Geometry check sheet. Reference: the model listing, model coordinates, mm. Face numbers are marked on the shaded views. Give positions to 0.01 mm unless a question says otherwise; leave off trailing zeros. Loops run counter-clockwise (first coordinate to the right, second up) from the corner with the lowest first, then second, coordinate; pieces in that order, holes last. Notation, with made-up numbers: (-31, 89) -> (26, 89) arc R25 ccw to (26, 119) -> close; hole circle Ø10 at (-3.75, 81). An arc over 180 degrees is marked (long way). Write item = value, one per line.
```python
from build123d import *

# Parameters (mm, degrees)
F1_DEPTH = 5.08
F0_W     = 32.385
F0_H     = 5.08
F2_DEPTH = 50.8
F3_DEPTH = 76.2
F4_DEPTH = 127
F5_R     = 2.53999


# Not quite as in the source:
# - a fillet or chamfer is up to 0.001 mm smaller than in the source, because OpenCascade refuses the exact size


with BuildPart() as f1:
    # F0 (on Top) → F1 (new body)
    with BuildSketch(Plane.XY):
        Polygon((23.8125, 15.24), (-23.8125, 15.24), (-23.8125, -15.24), (-16.1925, -15.24), (16.1925, -15.24), (23.8125, -15.24), align=None)
    extrude(amount=F1_DEPTH)

    # F0 (on Top) → F2 (join)
    with BuildSketch(Plane.XY):
        with Locations((0, -17.78)):
            Rectangle(F0_W, F0_H)
    extrude(amount=F2_DEPTH)

    # F0 (on Top) → F3 (join)
    with BuildSketch(Plane.XY):
        Polygon((-23.8125, 15.24), (-28.8925, 15.24), (-28.8925, -20.32), (-16.1925, -20.32), (-16.1925, -15.24), (-23.8125, -15.24), align=None)
        Polygon((28.8925, -20.32), (28.8925, 15.24), (23.8125, 15.24), (23.8125, -15.24), (16.1925, -15.24), (16.1925, -20.32), align=None)
    extrude(amount=F3_DEPTH)

    # F0 (on Top) → F4 (join)
    with BuildSketch(Plane.XY):
        Polygon((28.8925, 20.32), (-28.8925, 20.32), (-28.8925, 15.24), (-23.8125, 15.24), (23.8125, 15.24), (28.8925, 15.24), align=None)
    extrude(amount=F4_DEPTH)

    # F5 (radius 2.54 in the source; OpenCascade refuses exactly that, so slightly less here)
    f5_edges = [f1.edges().sort_by_distance(p)[0] for p in [
        (28.8925, -20.32, 38.1),
        (22.5425, -20.32, 76.2),
        (16.1925, -20.32, 63.5),
        (0, -20.32, 50.8),
        (-16.1925, -20.32, 63.5),
        (-22.5425, -20.32, 76.2),
        (-28.8925, -20.32, 38.1),
        (0, -20.32, 0),
        (-16.1925, -15.24, 63.5),
        (0, -15.24, 50.8),
        (-20.0025, -15.24, 76.2),
        (20.0025, -15.24, 76.2),
        (16.1925, -15.24, 63.5),
        (16.1925, -17.78, 76.2),
        (-16.1925, -17.78, 76.2),
        (23.8125, 0, 76.2),
        (-23.8125, 0, 76.2),
        (28.8925, -2.54, 76.2),
        (28.8925, 15.24, 101.6),
        (28.8925, 17.78, 127),
        (28.8925, 20.32, 63.5),
        (28.8925, 0, 0),
        (0, 15.24, 127),
        (-28.8925, 15.24, 101.6),
        (0, 20.32, 127),
        (-28.8925, 20.32, 63.5),
        (-28.8925, -2.54, 76.2),
        (-28.8925, 0, 0),
        (0, 20.32, 0),
        (-28.8925, 17.78, 127),
    ]]
    fillet(f5_edges, radius=F5_R)


solid = f1.part
```
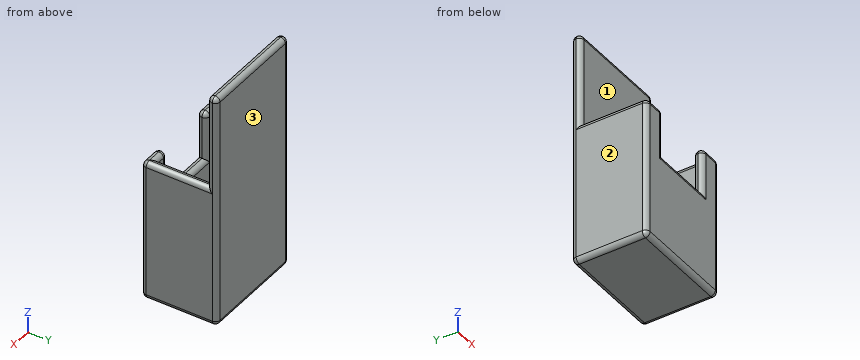
Item 1: Thickness scan on L1, parallel to Y at x = 15, z = 13; L2, parallel to X at y = 5, z = 55.5; L3, parallel to Z at x = -12, y = -14. Record the ranges inside material, lowest first. Write a range as [from, to].
Answer:
L1 = [-20.32, -15.24], [15.24, 20.32]
L2 = [-28.89, -23.81], [23.81, 28.89]
L3 = [0, 5.08]
Item 2: Draft check along X on the marked faces 1, 2 and 3. Enter one of: +X half, -X half, draft (parallel to the pull), parting line (faces both ways), or undercut.
Answer:
face_1 = undercut
face_2 = -X half
face_3 = draft
Item 3: Gauge pin test, flat ends, axial feed: pin 1 (4 mm diameter, centred on x = 23.5, y = -7.5, fed in from +Z); pin 2 (4 mm diameter, centred on x = -21.5, y = -7.5, fed in from +Z); pin 3 (10 mm diameter, centred on x = -1, z = 86, fed in from -Y). Record the tip position at first contact, or that the pin passes through.
Answer:
pin_1 = 76.05
pin_2 = 5.08
pin_3 = 15.24
Item 4: Section check A-A, the plane z = 43. Record the cut outline in (x, y), plus the area to 3 significant figures.
Answer:
outline = (-28.89, -17.78) arc R2.54 ccw to (-26.35, -20.32) -> (26.35, -20.32) arc R2.54 ccw to (28.89, -17.78) -> (28.89, 17.78) arc R2.54 ccw to (26.35, 20.32) -> (-26.35, 20.32) arc R2.54 ccw to (-28.89, 17.78) -> close; hole (-23.81, -15.24) -> (23.81, -15.24) -> (23.81, 15.24) -> (-23.81, 15.24) -> close
area = 891 mm^2
